from build123d import *

# Parameters (mm, degrees)
F0_W     = 59.436
F0_H     = 90.424
F1_DEPTH = 2.54
F2_R     = 2.286
F3_R     = 1.524
F4_R     = 1.778
F5_DEPTH = 25.4
F6_W     = 16.9672
F6_H     = 27.178
F7_DEPTH = 25.4


with BuildPart() as f1:
    # F0 (on Top) → F1 (new body)
    with BuildSketch(Plane.XY):
        Rectangle(F0_W, F0_H)
    extrude(amount=F1_DEPTH)

    # F2
    f2_edges = [f1.edges().sort_by_distance(p)[0] for p in [
        (29.718, -45.212, 1.27),
        (-29.718, -45.212, 1.27),
        (29.718, 45.212, 1.27),
        (-29.718, 45.212, 1.27),
    ]]
    fillet(f2_edges, radius=F2_R)

    # F3
    f3_edges = [f1.edges().sort_by_distance(p)[0] for p in [
        (-29.718, 0, 2.54),
    ]]
    fillet(f3_edges, radius=F3_R)

    # F4 (on face) → F5 (cut)
    with BuildSketch(Plane(origin=(0, 0, 0), x_dir=(1, 0, 0), z_dir=(0, 0, -1))):
        with Locations((0, 42.037)):
            Circle(F4_R)
        with Locations((0, -42.037)):
            Circle(F4_R)
    extrude(amount=-F5_DEPTH, mode=Mode.SUBTRACT)

    # F6 (on face) → F7 (cut)
    with BuildSketch(Plane.XY.offset(2.54)):
        with Locations((-0.922986, 4.603704)):
            Rectangle(F6_W, F6_H)
    extrude(amount=-F7_DEPTH, mode=Mode.SUBTRACT)


solid = f1.part
Check sheet for the modelled part. Datum: model origin and axes. Units: mm. A direction names the side the tool comes from. Round coordinates to 2 decimals unless told otherwise and drop trailing zeros. Loops run counter-clockwise (first coordinate to the right, second up) from the corner with the lowest first, then second, coordinate; pieces in that order, holes last. Notation, with made-up numbers: M -16,76 L 3,76 A16 cw 3,88 Z; hole C 43.25,57.25 d2. An arc over 180 degrees is marked long. One line per question, with ' | ' between items. Start each with the question number.
Item 1: Set-up check for faces 1 (the face through (7.561, 4, 1)), 2 (the face through (29.07, 44.52, 0.52)): record each of +Z, -Z, +X, -X, +Y, -Y from which the full face is reachable in a straight line by a thin tool's end or side.
Item 2: Gauge pin test, flat end, axial feed: pin 1 Ø3 at (x, y) = (0, 42.037) entering from +Z. Record the tip position at first contact, or that the pin passes through.
Item 3: Section check C-C (z = 1.7). State how many separate pieces and enclosed holes the cut face has, and give its area (3 significant figures).
Item 4: Section check A-A (y = 2). Record the boundary of the cut face in (x, z), and give its area (3 significant figures).
Item 5: Section check B-B (x = -6). Record the boundary of the cut face in (y, z).
Item 6: Scan lines: probe 1 along Y at (x, z) = (0, 1.15) (3 decimals); probe 2 along X at (y, z) = (-1, 2.3); probe 3 along Y at (x, z) = (0, 1.65) (3 decimals). Record each from-to range of solid material in increasing order.
Item 7: Release check for a two-part mould opening along Y. For faces 3 (the face through (-9.407, 4, 1)), 4 (the face through (12, 1, 2.54)), 5 (the face through (29.03, -44.56, 0.52)) record: released by +Y, released by -Y, zero draft, split by the parting line, or undercut.
Worked out:
1) face 1: +Z, -Z | face 2: +Z, -Z, +X, +Y
2) pin 1: through
3) separate pieces: 1 | enclosed holes: 3 | area: 4,840 mm^2
4) outline: M -29.72,0 L -9.41,0 L -9.41,2.54 L -28.19,2.54 A1.52 ccw -29.72,1.02 Z; M 7.56,0 L 29.72,0 L 29.72,1.02 A1.52 ccw 28.19,2.54 L 7.56,2.54 Z | area: 107 mm^2
5) outline: M -45.21,0 L -8.99,0 L -8.99,2.54 L -43.69,2.54 A1.52 ccw -45.21,1.02 Z; M 18.19,0 L 45.21,0 L 45.21,1.02 A1.52 ccw 43.69,2.54 L 18.19,2.54 Z
6) probe 1: -45.206 to -43.815, -40.259 to -8.985, 18.193 to 40.259, 43.815 to 45.206 | probe 2: -29.01 to -9.41, 7.56 to 29.01 | probe 3: -45.074 to -43.815, -40.259 to -8.985, 18.193 to 40.259, 43.815 to 45.074
7) face 3: undercut | face 4: zero draft | face 5: released by -Y
